```python
from build123d import *

# Parameters (mm, degrees)
SKETCH1_R           = 22.5
BOSS_EXTRUDE1_DEPTH = 3
SKETCH2_R           = 5
BOSS_EXTRUDE2_DEPTH = 70
SKETCH3_R           = 12
BOSS_EXTRUDE3_DEPTH = 28
FILLET1_R           = 6
SKETCH4_W           = 14.522746449
SKETCH4_H           = 20
CUT_EXTRUDE2_DEPTH  = 14
SKETCH5_R           = 4
CUT_EXTRUDE3_DEPTH  = 31
SKETCH7_R           = 9
SKETCH7_R_2         = 4
BOSS_EXTRUDE4_DEPTH = 12.5


with BuildPart() as part:
    # Sketch1 → Boss-Extrude1 (new body)
    with BuildSketch(Plane(origin=(0, 0, 0), x_dir=(1, 0, 0), z_dir=(0, 1, 0))):
        Circle(SKETCH1_R)
    extrude(amount=BOSS_EXTRUDE1_DEPTH)

    # Sketch2 → Boss-Extrude2 (add)
    with BuildSketch(Plane(origin=(0, 3, 0), x_dir=(1, 0, 0), z_dir=(0, 1, 0))):
        Circle(SKETCH2_R)
    extrude(amount=BOSS_EXTRUDE2_DEPTH)

    # Sketch3 → Boss-Extrude3 (add)
    with BuildSketch(Plane.XZ):
        Circle(SKETCH3_R)
    extrude(amount=BOSS_EXTRUDE3_DEPTH)

    # Fillet1
    fillet1_edges = [part.edges().sort_by_distance(p)[0] for p in [
        (-12, -28, 0),
    ]]
    fillet(fillet1_edges, radius=FILLET1_R)

    # Sketch4 → Cut-Extrude2 (cut, symmetric)
    with BuildSketch(Plane.XY):
        with Locations((-14.761373225, -18)):
            Rectangle(SKETCH4_W, SKETCH4_H)
        with Locations((14.761373225, -18)):
            Rectangle(SKETCH4_W, SKETCH4_H)
    extrude(amount=CUT_EXTRUDE2_DEPTH, both=True, mode=Mode.SUBTRACT)

    # Sketch5 → Cut-Extrude3 (cut, through all)
    with BuildSketch(Plane(origin=(7.5, 0, 0), x_dir=(0, 0, -1), z_dir=(1, 0, 0))):
        with Locations((0, -18)):
            Circle(SKETCH5_R)
    extrude(amount=-CUT_EXTRUDE3_DEPTH, mode=Mode.SUBTRACT)

    # Sketch7 → Boss-Extrude4 (add, symmetric)
    with BuildSketch(Plane(origin=(0, 0, 0), x_dir=(0, 0, -1), z_dir=(1, 0, 0))):
        with Locations((0, -18)):
            Circle(SKETCH7_R)
        with Locations((0, -18)):
            Circle(SKETCH7_R_2, mode=Mode.SUBTRACT)
    extrude(amount=BOSS_EXTRUDE4_DEPTH, both=True)


solid = part.part
```
Build history of the part. All positions in model axes, mm. A direction names the side the tool comes from. Round coordinates to 2 decimals unless told otherwise and drop trailing zeros. Write each loop counter-clockwise with the first axis right and the second up, starting at its lowest first coordinate (ties: lowest second). Pieces come first, ordered by that corner, then holes.
1) Drill centre lines: probe 1 along Y at (x, z) = (1, 0); probe 2 along Y at (x, z) = (9.5, 2.5); probe 3 along Y at (x, z) = (12, -1). Where is each one in solid material? Low to high.
2) 3-axis set-ups, long thin cutter, end or side, ignore diameter. For faces 1 (the flat face through (7.5, -9, -2)), 2 (the flat face through (-12.5, -22, -2)), 3 (the cylindrical face through (-1.08, 37.51, 4.88)), 4 (the flat face through (-7.5, -9, 2)), 5 (the flat face through (9, -8, 0)): which of +Z, -Z, +X, -X, +Y, -Y reach the whole face in a straight line?
3) Pin check, flat tips, straight feed: pin 1 (8 mm diameter, centred on y = 58, z = 0, fed in from +X); pin 2 (5.5 mm diameter, centred on y = -15.5, z = -3.5, fed in from -X); pin 3 (5 mm diameter, centred on x = -15.5, z = 11, fed in from +Y). Stop position of each tip, or through.
4) Mould opens along Y. For faces 6 (the flat face through (0, 73, 0)), 7 (the flat face through (12.5, -22, -2)), 8 (the cylindrical face through (11.446, -5.957, 3.604)), 9 (the flat face through (0, -28, 0)) say: +Y half, -Y half, draft (parallel to the pull), parting line (faces both ways), or undercut.
5) Band-saw the part on B-B, the plane x = -9.5. List the corners of the cut face in (y, z).
6) Band-saw the part on A-A, the plane y = -18. List the corners of the cut face in (x, z).
7) Band-saw the part on D-D, the plane z = 15.5. List the corners of the cut face in (x, y), and give its area (3 significant figures).
8) Band-saw the part on C-C, the plane x = -18. List the corners of the cut face in (y, z).
Ans:
1. probe 1: y = -28 to -22, -14 to 73
1. probe 2: y = -26.65 to -21.12, -14.88 to -9.35, -8 to 3
1. probe 3: y = -26.94 to -21.87, -14.13 to -9.06, 0 to 3
2. face 1: +X
2. face 2: +Z, -Z, -X, -Y
2. face 3: +Y
2. face 4: -X
2. face 5: +Z, -Z, +X
3. pin 1: stops at x = 5
3. pin 2: stops at x = -12.5
3. pin 3: stops at y = 3
4. face 6: +Y half
4. face 7: draft
4. face 8: undercut
4. face 9: -Y half
5. outline: circle Ø18 at (-18, 0); (-8, -7.33) - (0, -7.33) - (0, -20.4) - (3, -20.4) - (3, 20.4) - (0, 20.4) - (0, 7.33) - (-8, 7.33) - close; hole circle Ø8 at (-18, 0)
6. outline: (-12.5, -9) - (-7.5, -9) - (-7.5, -9.37) arc R12 ccw to (7.5, -9.37) - (7.5, -9) - (12.5, -9) - (12.5, -4) - (-12.5, -4) - close; (-12.5, 4) - (12.5, 4) - (12.5, 9) - (7.5, 9) - (7.5, 9.37) arc R12 ccw to (-7.5, 9.37) - (-7.5, 9) - (-12.5, 9) - close
7. outline: (-16.31, 0) - (16.31, 0) - (16.31, 3) - (-16.31, 3) - close
7. area: 97.9 mm2
8. outline: (0, -13.5) - (3, -13.5) - (3, 13.5) - (0, 13.5) - close
